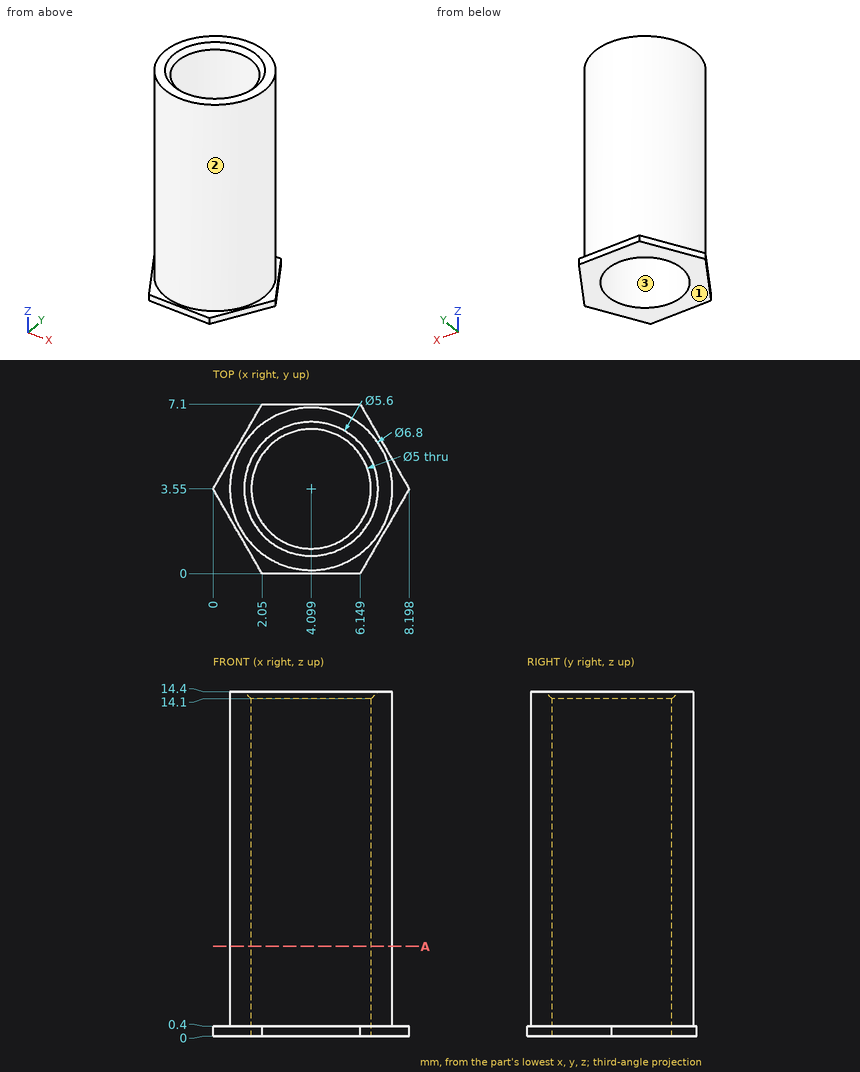
Can you work these out from the drawing? Everything is in mm from the part's minimum corner. Give positions to 0.01 mm unless a question says otherwise; leave off trailing zeros. Order: outer loops, then holes, each group sorted by start corner. A loop starts at its lowest first (then second) coordinate and runs counter-clockwise, first axis right, second up. Notation, with made-up numbers: M -25,80.25 L -21,80.25 A10 ccw -21,84.25 Z; hole C 3.25,36 d2. An arc over 180 degrees is marked long. One line per item, written item: value.
Item 1: For pin 1 (2 mm diameter, centred on x = 3.5, z = 2, fed in from +Y); pin 2 (3 mm diameter, centred on y = 1.5, z = 5.5, fed in from +X) (1 decimal); pin 3 (2 mm diameter, centred on x = 5.5, z = 5.5, fed in from -Y), each with a flat end and sliding along its axis, tell me the tip position at first contact or that it passes through.
Verdict:
pin 1: y = 6.95
pin 2: x = 7.5
pin 3: y = 0.17
Item 2: If we mould it in two halves opening along Y, with no side actions, what happens to the marked faces 1, 2 and 3? For each: pulls with the +Y half, pulls with the -Y half, needs draft (parallel to the pull), parting line crosses it, or undercut.
Verdict:
face 1: needs draft
face 2: parting line crosses it
face 3: undercut
Item 3: If we section it at A-A on z = 3.75: Write out the boundary of the cut face in (x, y).
Verdict:
outline: C 4.1,3.55 d6.8; hole C 4.1,3.55 d5
Item 4: Please list where these lines run through material, in increasing order: line 1 (X direction, y = 1.5, z = 10.5) (1 decimal); line 2 (Y direction, x = 2.5, z = 5.5); line 3 (X direction, y = 3.75, z = 8.5) (1 decimal).
Verdict:
line 1: 1.4 to 2.7, 5.5 to 6.8
line 2: 0.55 to 1.63, 5.47 to 6.55
line 3: 0.7 to 1.6, 6.6 to 7.5
